Read the model definition and answer for the solid it produces. Units are mm, in the model's axes. A direction names the side the tool comes from. Give positions to 0.01 mm unless a question says otherwise; leave off trailing zeros. Order: outer loops, then holes, each group sorted by start corner. A loop starts at its lowest first (then second) coordinate and runs counter-clockwise, first axis right, second up. Notation, with made-up numbers: (35.25, 9) - (43.25, 9) arc R8 cw to (43.25, 24) - close; hole circle Ø9 at (-2, 39). An arc over 180 degrees is marked (long way). Write each question's results on one line, items separated by ' | '. Start each with the question number.
Q1. Find section D-D on z = -113. Give the vertices of the cut face in (x, y).
Q2. Flat-ended cylindrical pins translate along their axes: P1, Ø8, axis at x = 28.3, z = -267.29, coming from the -Y side; P2, Ø4, axis at x = 262, y = 3, coming from the -Z side; P3, Ø4, axis at x = 226.5, y = 2.5, coming from the -Z side; P4, Ø2, axis at y = 1, z = 8, coming from the +X side. Find the tip coordinate at first contact, or state that the pin passes through.
Q3. Find section B-B on y = 3.25. Count the separate pieces of the cut face and the enclosed holes in it, and give its area (3 significant figures).
Q4. Find the intervals of material crossed by line 1 along X through (y, z) = (1, -293.5); line 2 along Z through (x, y) = (267.5, 4.25); line 3 along X through (y, z) = (4, 32), in increasing order. Write a range as from..to.
Q5. For a pull along Z with two mould halves and no side action, classify faces 1 (the face through (141, 0, -153)), 2 (the face through (229.65, 3.51, -17.37)), 3 (the face through (303.46, 3.51, 10.78)) as +Z half, -Z half, draft (parallel to the pull), parting line (faces both ways), or undercut.
Q6. Find section A-A on x = 216. Give the vertices of the cut face in (y, z).
Q7. A tool of negligible diameter and unlimited length cuts with its end or side. For faces 4 (the face through (262.03, 3.51, -49.75)), 5 (the face through (264.902, 3.506, -254.845)), 6 (the face through (17.37, 3.51, -49.75)), 7 (the face through (49.75, 3.51, -17.37)), from which of +Z, -Z, +X, -X, +Y, -Y can it reach the whole face along a straight path? Write none if from no direction.
Q8. Find section C-C on x = 151. Give the vertices of the cut face in (y, z).
Autodesk Inventor part; units mm, degrees
ref_plane "YZ Plane" through (0, 0, 0) normal (1, 0, 0) x (0, 1, 0)
ref_plane "XZ Plane" through (0, 0, 0) normal (0, 1, 0) x (-1, 0, 0)
ref_plane "XY Plane" through (0, 0, 0) normal (0, 0, 1) x (1, 0, 0)
sketch "Sketch1" plane through (0, 0, 0) normal (0, 1, 0) x (-1, 0, 0)
  line L0 (-16.1896, 16.1896) -> (10.7512, 43.1304)
  line L1 (-295.5896, -16.1896) -> (-322.5304, 10.7512)
  line L2 (16.1896, -263.2104) -> (43.1304, -290.1512)
  line L3 (-43.1304, -268.6488) -> (10.7512, -322.5304)
  line L4 (-10.7512, -236.2696) -> (16.1896, -263.2104)
  line L5 (-295.5896, -263.2104) -> (-268.6488, -236.2696)
  line L6 (-290.1512, -322.5304) -> (-236.2696, -268.6488)
  line L7 (-322.5304, -290.1512) -> (-295.5896, -263.2104)
  arc A0 (-290.1512, 43.1304) -> (-322.5304, 10.7512) centre (-306.3408, 26.9408) ccw
  arc A1 (-322.5304, -290.1512) -> (-290.1512, -322.5304) centre (-306.3408, -306.3408) ccw
  arc A2 (10.7512, -322.5304) -> (43.1304, -290.1512) centre (26.9408, -306.3408) ccw
  arc A3 (43.1304, 10.7512) -> (10.7512, 43.1304) centre (26.9408, 26.9408) ccw
  line L8 (-329.2363, 49.8363) -> (49.8363, 49.8363)
  line L9 (49.8363, -329.2363) -> (49.8363, 49.8363)
  line L10 (49.8363, -329.2363) -> (-329.2363, -329.2363)
  line L11 (-329.2363, 49.8363) -> (-329.2363, -329.2363)
  line L12 (-10.7512, -236.2696) -> (-76.2, -170.8208)
  line L13 (-170.8208, -76.2) -> (-290.1512, 43.1304)
  line L14 (-43.1304, -268.6488) -> (-108.5792, -203.2)
  line L15 (-203.2, -108.5792) -> (-295.5896, -16.1896)
  line L16 (-236.2696, -268.6488) -> (-170.8208, -203.2)
  line L17 (-76.2, -108.5792) -> (43.1304, 10.7512)
  line L18 (-268.6488, -236.2696) -> (-203.2, -170.8208)
  line L19 (-108.5792, -76.2) -> (-16.1896, 16.1896)
  line L20 (-108.5792, -76.2) -> (-170.8208, -76.2)
  line L21 (-203.2, -108.5792) -> (-203.2, -170.8208)
  line L22 (-170.8208, -203.2) -> (-108.5792, -203.2)
  line L23 (-76.2, -170.8208) -> (-76.2, -108.5792)
  circle A4 centre (2254.858, -433.3281) radius 4.2386
  circle A5 centre (2254.858, -433.3281) radius 14.0056
  line L24 (2254.858, -433.3281) -> (2238.6684, -449.5177)
  line L25 (2254.858, -433.3281) -> (2271.0476, -417.1385)
  line L26 (2238.6684, -449.5177) -> (2211.7277, -422.5769)
  line L27 (2271.0476, -417.1385) -> (2297.9884, -444.0792)
  line L28 (2211.7277, -422.5769) -> (2265.6092, -476.4584)
  line L29 (2265.6092, -476.4584) -> (2297.9884, -444.0792)
  line L30 (2297.9884, -444.0792) -> (2244.1069, -390.1977)
  line L31 (2244.1069, -390.1977) -> (2211.7277, -422.5769)
  line L32 (-29.66, -282.1192) -> (-43.1304, -268.6488)
  line L33 (-43.1304, -268.6488) -> (-29.66, -282.1192)
  line L34 (2.7192, -249.74) -> (-10.7512, -236.2696)
  line L35 (-10.7512, -236.2696) -> (-43.1304, -268.6488)
  line L36 (-43.1304, -268.6488) -> (-29.66, -282.1192)
  line L37 (-29.66, -282.1192) -> (2.7192, -249.74)
  line L38 (-43.1304, -268.6488) -> (-36.3952, -275.384)
  circle A6 centre (-28.2995, -267.2883) radius 4.445
  circle A7 centre (-12.1081, -251.0969) radius 4.445
  line L39 (10.7512, -322.5304) -> (43.1304, -290.1512)
  circle A8 centre (28.3031, -291.5081) radius 4.445
  line L40 (43.1304, -290.1512) -> (29.66, -276.6808)
  line L41 (29.66, -276.6808) -> (-2.7192, -309.06)
  line L42 (29.66, -276.6808) -> (-2.7192, -309.06)
  circle A9 centre (12.1117, -307.6995) radius 4.445
  line L43 (10.7512, -322.5304) -> (-2.7192, -309.06)
  line L44 (-2.7192, -309.06) -> (10.7512, -322.5304)
  line L45 (-2.7192, -309.06) -> (4.016, -315.7952)
  line L46 (-2.7192, -309.06) -> (10.7512, -322.5304)
  line L47 (-76.2, -170.8208) -> (-114.6919, -170.8208)
  circle A10 centre (-279.4, 0) radius 4.2386
  circle A11 centre (-279.4, 0) radius 14.0056
  line L48 (-322.5304, 10.7512) -> (-268.6488, -43.1304)
  line L49 (-236.2696, -10.7512) -> (-290.1512, 43.1304)
  line L50 (-268.6488, -43.1304) -> (-236.2696, -10.7512)
  line L51 (-263.2104, 16.1896) -> (-236.2696, -10.7512)
  line L52 (-279.4, 0) -> (-295.5896, -16.1896)
  line L53 (-279.4, 0) -> (-263.2104, 16.1896)
  circle A12 centre (-291.5081, 28.3031) radius 4.445
  line L54 (-309.06, -2.7192) -> (-276.6808, 29.66)
  line L55 (-276.6808, 29.66) -> (-290.1512, 43.1304)
  line L56 (-290.1512, 43.1304) -> (-322.5304, 10.7512)
  line L57 (-290.1512, 43.1304) -> (-322.5304, 10.7512)
  circle A13 centre (-307.6995, 12.1117) radius 4.445
  line L58 (-295.5896, -16.1896) -> (-322.5304, 10.7512)
  line L59 (-309.06, -2.7192) -> (-322.5304, 10.7512)
  line L60 (-322.5304, 10.7512) -> (-309.06, -2.7192)
  line L61 (-322.5304, 10.7512) -> (-309.06, -2.7192)
  line L62 (-322.5304, 10.7512) -> (-315.7952, 4.016)
  circle A14 centre (-251.0969, -12.1081) radius 4.445
  line L63 (-249.74, 2.7192) -> (-282.1192, -29.66)
  line L64 (-249.74, 2.7192) -> (-282.1192, -29.66)
  line L65 (-282.1192, -29.66) -> (-275.384, -36.3952)
  circle A15 centre (-267.2883, -28.2995) radius 4.445
  line L66 (-268.6488, -43.1304) -> (-236.2696, -10.7512)
  line L67 (-268.6488, -43.1304) -> (-282.1192, -29.66)
  line L68 (-282.1192, -29.66) -> (-268.6488, -43.1304)
  line L69 (-282.1192, -29.66) -> (-268.6488, -43.1304)
  line L70 (-236.2696, -10.7512) -> (-249.74, 2.7192)
  circle A16 centre (0, 0) radius 4.2386
  circle A17 centre (0, 0) radius 14.0056
  line L71 (-10.7512, -43.1304) -> (43.1304, 10.7512)
  line L72 (10.7512, 43.1304) -> (-43.1304, -10.7512)
  line L73 (43.1304, 10.7512) -> (10.7512, 43.1304)
  line L74 (-16.1896, 16.1896) -> (10.7512, 43.1304)
  line L75 (0, 0) -> (16.1896, -16.1896)
  line L76 (0, 0) -> (-16.1896, 16.1896)
  circle A18 centre (-28.3031, -12.1081) radius 4.445
  line L77 (2.7192, -29.66) -> (-29.66, 2.7192)
  line L78 (-29.66, 2.7192) -> (-43.1304, -10.7512)
  line L79 (-43.1304, -10.7512) -> (-10.7512, -43.1304)
  line L80 (-43.1304, -10.7512) -> (-10.7512, -43.1304)
  circle A19 centre (-12.1117, -28.2995) radius 4.445
  line L81 (16.1896, -16.1896) -> (-10.7512, -43.1304)
  line L82 (2.7192, -29.66) -> (-10.7512, -43.1304)
  line L83 (-10.7512, -43.1304) -> (2.7192, -29.66)
  line L84 (-10.7512, -43.1304) -> (2.7192, -29.66)
  line L85 (-10.7512, -43.1304) -> (-4.016, -36.3952)
  circle A20 centre (12.1081, 28.3031) radius 4.445
  line L86 (-2.7192, 29.66) -> (29.66, -2.7192)
  line L87 (-2.7192, 29.66) -> (29.66, -2.7192)
  line L88 (29.66, -2.7192) -> (36.3952, 4.016)
  circle A21 centre (28.2995, 12.1117) radius 4.445
  line L89 (43.1304, 10.7512) -> (10.7512, 43.1304)
  line L90 (43.1304, 10.7512) -> (29.66, -2.7192)
  line L91 (29.66, -2.7192) -> (43.1304, 10.7512)
  line L92 (29.66, -2.7192) -> (43.1304, 10.7512)
  line L93 (10.7512, 43.1304) -> (-2.7192, 29.66)
  circle A22 centre (-291.5117, -307.6995) radius 4.445
  circle A23 centre (-307.7031, -291.5081) radius 4.445
  line L94 (-309.06, -276.6808) -> (-322.5304, -290.1512)
  line L95 (-276.6808, -309.06) -> (-290.1512, -322.5304)
  line L96 (-290.1512, -322.5304) -> (-276.6808, -309.06)
  line L97 (-290.1512, -322.5304) -> (-276.6808, -309.06)
  line L98 (-263.2104, -295.5896) -> (-290.1512, -322.5304)
  line L99 (-268.6488, -236.2696) -> (-322.5304, -290.1512)
  line L100 (-290.1512, -322.5304) -> (-236.2696, -268.6488)
  line L101 (-290.1512, -322.5304) -> (-283.416, -315.7952)
  line L102 (-268.6488, -236.2696) -> (-282.1192, -249.74)
  circle A24 centre (-267.2919, -251.0969) radius 4.445
  line L103 (-295.5896, -263.2104) -> (-268.6488, -236.2696)
  circle A25 centre (-251.1005, -267.2883) radius 4.445
  line L104 (-249.74, -282.1192) -> (-243.0048, -275.384)
  line L105 (-249.74, -282.1192) -> (-236.2696, -268.6488)
  line L106 (-249.74, -282.1192) -> (-236.2696, -268.6488)
  line L107 (-236.2696, -268.6488) -> (-249.74, -282.1192)
  line L108 (-290.1512, -322.5304) -> (-322.5304, -290.1512)
  point P0 (-279.4, 0)
  point P1 (-279.4, -279.4)
  dimension "d68" = 379.0727
  dimension "d69" = 379.0727
  dimension "d70" = 379.0727
  dimension "d77" = 45.7911
  dimension "d78" = 8.4772
  dimension "d79" = 28.0111
  dimension "d80" = 22.8956
  dimension "d81" = 22.8956
  dimension "d82" = 38.1
  dimension "d83" = 38.1
  dimension "d84" = 45.7962
  dimension "d85" = 76.2
  dimension "d86" = 45.7911
  dimension "d87" = 19.05
  dimension "d88" = 19.05
  dimension "d89" = 9.525
  dimension "d90" = 8.89
  dimension "d91" = 45.7911
  dimension "d92" = 45.7911
  dimension "d93" = 19.05
  dimension "d94" = 19.05
  dimension "d95" = 9.525
  dimension "d96" = 8.89
  dimension "d97" = 135
  dimension "d98" = 8.4772
  dimension "d99" = 28.0111
  dimension "d100" = 22.8956
  dimension "d101" = 22.8956
  dimension "d102" = 38.1
  dimension "d103" = 38.1
  dimension "d104" = 45.7911
  dimension "d105" = 76.2
  dimension "d106" = 45.7911
  dimension "d107" = 19.05
  dimension "d108" = 19.05
  dimension "d109" = 9.525
  dimension "d110" = 8.89
  dimension "d111" = 45.7911
  dimension "d112" = 45.7911
  dimension "d113" = 19.05
  dimension "d114" = 19.05
  dimension "d115" = 9.525
  dimension "d116" = 8.89
  dimension "d117" = 8.4772
  dimension "d118" = 28.0111
  dimension "d119" = 22.8956
  dimension "d120" = 22.8956
  dimension "d121" = 38.1
  dimension "d122" = 38.1
  dimension "d123" = 45.7962
  dimension "d124" = 76.2
  dimension "d125" = 45.7911
  dimension "d126" = 19.05
  dimension "d127" = 19.05
  dimension "d128" = 9.525
  dimension "d129" = 8.89
  dimension "d130" = 45.7911
  dimension "d131" = 45.7911
  dimension "d132" = 19.05
  dimension "d133" = 19.05
  dimension "d134" = 9.525
  dimension "d135" = 8.89
  dimension "d140" = 38.1
  dimension "d141" = 38.1
extrude "Extrusion2" add sketch "Sketch1" along normal blind 7.112 contours L76 A17 L75 L17 L77 L19 | L0 L86 L17 L75 A17 L76 | L0 L73 L17 L86 | L77 L17 L79 L19 | L76 A16 L75 A17 | A17 L75 A16 L76 | A3 L73 | L79 L17 L23 L12 L35 L14 L22 L16 L6 L108 L7 L5 L18 L21 L15 L50 L13 L20 L19 | L76 L75 A16 | A16 L75 L76 | A0 L56 | A2 L39 | L13 L54 L1 L56 | L50 L15 L63 L13 | L39 L3 L41 L2 | L13 L53 A11 L52 L1 L54 | A1 L108 | L63 L15 L52 A11 L53 L13 | L4 L37 L3 L35 | L41 L3 L37 L4 L2 | L53 A10 L52 A11 | A11 L52 A10 L53 | L53 L52 A10 | A10 L52 L53
properties part number "drone frame"
Working result:
1) outline: (76.2, 0) - (203.2, 0) - (203.2, 7.11) - (76.2, 7.11) - close
2) P1: through | P2: z = -296.38 | P3: z = -260.88 | P4: x = 320.78
3) separate pieces: 1 | enclosed holes: 16 | area: 47,200 mm²
4) line 1: -45.9..-32.28, -24.33..18.28, 261.12..303.73, 311.68..325.3 | line 2: -299.88..-255.54, -246.66..-235.12, -44.28..-32.74, -23.86..20.48 | line 3: -49.27..-14.58, -9.64..0.38, 279.02..289.04, 293.98..328.67
5) face 1: draft | face 2: +Z half | face 3: undercut
6) outline: (0, -248.38) - (7.11, -248.38) - (7.11, -183.62) - (0, -183.62) - close; (0, -95.78) - (7.11, -95.78) - (7.11, -31.02) - (0, -31.02) - close
7) face 4: +X, +Y, -Y | face 5: +Y, -Y | face 6: -X, +Y, -Y | face 7: +Z, +Y, -Y
8) outline: (0, -203.2) - (7.11, -203.2) - (7.11, -76.2) - (0, -76.2) - close
